```python
from build123d import *

# Parameters (mm, degrees)
SKETCH1_R             = 1.7
SKETCH1_R_2           = 1.25
BOSS_EXTRUDE1_DEPTH   = 5
SKETCH11_W            = 16
SKETCH11_H            = 16
CUT_EXTRUDE6_DEPTH    = 4
SKETCH13_W            = 7.423787947
SKETCH13_H            = 16.529940363
CUT_EXTRUDE8_DEPTH    = 1
CHAMFER2_SIZE2        = 1
CHAMFER2_SIZE         = 0.707106781
CHAMFER2_EDGE_2_SIZE2 = 1
CHAMFER2_EDGE_2_SIZE  = 0.707106781
CHAMFER2_EDGE_3_SIZE2 = 1
CHAMFER2_EDGE_3_SIZE  = 0.707106781
CHAMFER2_EDGE_4_SIZE2 = 0.707106781
CHAMFER2_EDGE_4_SIZE  = 1
SKETCH15_R            = 1.7
CUT_EXTRUDE9_DEPTH    = 5


with BuildPart() as part:
    # Sketch1 → Boss-Extrude1 (new body)
    with BuildSketch(Plane.XY):
        Polygon((0, -8), (-16, -8), (-19, -5), (-20.515302869, -5), (-21.413786532, -4.101516338), (-21.413786532, -1.535700598), (-21.413786532, 4.101516338), (-20.515302869, 5), (-19, 5), (-16, 8), (0, 8), (3.535533906, 4.464466094), (6, 4.464466094), (7.7, 4.464466094), (9.467766953, 2.696699141), (9.467766953, -2.696699141), (7.7, -4.464466094), (6, -4.464466094), (3.535533906, -4.464466094), align=None)
        with Locations((6, 0)):
            Circle(SKETCH1_R, mode=Mode.SUBTRACT)
        with Locations((-19, 0)):
            Circle(SKETCH1_R_2, mode=Mode.SUBTRACT)
    extrude(amount=BOSS_EXTRUDE1_DEPTH)

    # Sketch11 → Cut-Extrude6 (cut)
    with BuildSketch(Plane.XY.offset(5)):
        with Locations((-8, 0)):
            Rectangle(SKETCH11_W, SKETCH11_H)
    extrude(amount=-CUT_EXTRUDE6_DEPTH, mode=Mode.SUBTRACT)

    # Sketch13 → Cut-Extrude8 (cut)
    with BuildSketch(Plane.XY.offset(5)):
        with Locations((-19.711893974, -0.264970181)):
            Rectangle(SKETCH13_W, SKETCH13_H)
    extrude(amount=-CUT_EXTRUDE8_DEPTH, mode=Mode.SUBTRACT)

    # Chamfer2
    chamfer2_edges = [part.edges().sort_by_distance(p)[0] for p in [
        (0, -8, 3),
    ]]
    chamfer(chamfer2_edges, length=CHAMFER2_SIZE, length2=CHAMFER2_SIZE2)

    # Chamfer2 edge 2
    chamfer2_edge_2_edges = [part.edges().sort_by_distance(p)[0] for p in [
        (0, 8, 3),
    ]]
    chamfer(chamfer2_edge_2_edges, length=CHAMFER2_EDGE_2_SIZE, length2=CHAMFER2_EDGE_2_SIZE2)

    # Chamfer2 edge 3
    chamfer2_edge_3_edges = [part.edges().sort_by_distance(p)[0] for p in [
        (-16, -8, 2.5),
    ]]
    chamfer(chamfer2_edge_3_edges, length=CHAMFER2_EDGE_3_SIZE, length2=CHAMFER2_EDGE_3_SIZE2)

    # Chamfer2 edge 4
    chamfer2_edge_4_edges = [part.edges().sort_by_distance(p)[0] for p in [
        (-16, 8, 2.5),
    ]]
    chamfer(chamfer2_edge_4_edges, length=CHAMFER2_EDGE_4_SIZE, length2=CHAMFER2_EDGE_4_SIZE2)

    # Mirror1: part across plane


with BuildPart() as part_1:
    add(part.part)
    add(part.part.mirror(Plane(origin=(0, 0, 5), x_dir=(1, 0, 0), z_dir=(0, 0, -1))))

    # Sketch15 → Cut-Extrude9 (cut)
    with BuildSketch(Plane.XY.offset(10)):
        with Locations((-19, 0)):
            Circle(SKETCH15_R)
    extrude(amount=-CUT_EXTRUDE9_DEPTH, mode=Mode.SUBTRACT)


solid = part_1.part
```
Source: CAD feature listing. Evaluate the final solid. Frame: model axes, mm. A direction names the side the tool comes from. Round coordinates to 2 decimals unless told otherwise and drop trailing zeros. Write each loop counter-clockwise with the first axis right and the second up, starting at its lowest first coordinate (ties: lowest second). Pieces come first, ordered by that corner, then holes. Notation, with made-up numbers: M 65,-37.75 L 86,-37.75 A10 cw 86,-28.75 Z; hole C -8.75,86 d4. An arc over 180 degrees is marked long. Answer as a JSON object with one key per item and string values. Group by question number.
(1) Section query C-C on x = -2. Output: boundary loops of the cut face in (y, z).
(2) Section query D-D on y = -6.5. Output: boundary loops of the cut face in (x, z).
(3) Section query A-A on z = 7. Output: boundary loops of the cut face in (x, y).
(4) Mould query, pull axis Y, two halves, no side actions, for faces 4 (the cylindrical face through (-17.43, -0.65, 8.03)), 5 (the flat face through (-17.5, 0.2, 4)), 6 (the flat face through (-20, 5, 2)). Classes: +Y half, -Y half, draft (parallel to the pull), parting line (faces both ways), or undercut.
(5) Ray query, line 1 (Z direction, x = -10, y = 1); line 2 (X direction, y = 2, z = 8.5); line 3 (Y direction, x = -19, z = 8.35). Return the intervals inside material, ascending. Write a range as [from, to].
(6) Reachability of faces 1 (the flat face through (-17, 0, 6)), 2 (the flat face through (0, 0, 5)), 3 (the flat face through (-20, -5, 2)) from +Z, -Z, +X, -X, +Y, -Y: full face, straight path, thin tool, end or side. Return the list, or none.
(7) First-contact query: pin 1 (4 mm diameter, centred on x = -19, y = 0, fed in from -Z); pin 2 (0.8 mm diameter, centred on x = -19.5, z = 8.5, fed in from -Y); pin 3 (5 mm diameter, centred on y = 5.5, z = 3.5, fed in from +X); pin 4 (0.9 mm diameter, centred on y = -3.5, z = 3, fed in from +X). Flat tips, straight axial feed; report the tip coordinate or a pass-through.
(8) Section query B-B on y = 0. Output: boundary loops of the cut face in (x, z), then the cut area to 3 significant figures.
Computed values:
{
 "1": {"outline": "M -8,0 L 8,0 L 8,1 L -8,1 Z; M -8,9 L 8,9 L 8,10 L -8,10 Z"},
 "2": {"outline": "M -17.5,0 L 1.5,0 L 1.5,10 L -17.5,10 L -17.5,6 L -16,6 L -16,9 L 0,9 L 0,1 L -16,1 L -16,4 L -17.5,4 Z"},
 "3": {"outline": "M -21.41,-4.1 L -20.52,-5 L -19,-5 L -16.71,-7.29 L -16,-7.29 L -16,7 L -16.5,7.5 L -19,5 L -20.52,5 L -21.41,4.1 Z; M 0,-7 L 0.5,-7.5 L 3.54,-4.46 L 7.7,-4.46 L 9.47,-2.7 L 9.47,2.7 L 7.7,4.46 L 3.54,4.46 L 0.71,7.29 L 0,7.29 Z; hole C -19,0 d3.4; hole C 6,0 d3.4"},
 "4": {"face 4": "undercut", "face 5": "draft", "face 6": "+Y half"},
 "5": {"line 1": "[0, 1], [9, 10]", "line 2": "[-21.41, -16], [0, 9.47]", "line 3": "[-5, -1.7], [1.7, 5]"},
 "6": {"face 1": "-X, +Y, -Y", "face 2": "+Y, -Y", "face 3": "+Z, -Z, -X, -Y"},
 "7": {"pin 1": "z = 0", "pin 2": "y = -5", "pin 3": "x = 9.16", "pin 4": "x = 9.11"},
 "8": {"outline": "M -21.41,0 L -20.25,0 L -20.25,4 L -21.41,4 Z; M -21.41,6 L -20.7,6 L -20.7,10 L -21.41,10 Z; M -17.75,0 L 4.3,0 L 4.3,10 L -17.3,10 L -17.3,6 L -16,6 L -16,9 L 0,9 L 0,1 L -16,1 L -16,4 L -17.75,4 Z; M 7.7,0 L 9.47,0 L 9.47,10 L 7.7,10 Z", "area": "112 mm^2"}
}
